from build123d import *

# Parameters (mm, degrees)
F0_W      = 90
F0_H      = 130
F1_DEPTH  = 20
F2_W      = 50
F2_H      = 2
F3_DEPTH  = 40
F4_W      = 50
F4_H      = 45
F5_DEPTH  = 2
F6_T      = -2
F7_R      = 2
F8_R      = 2
F9_R      = 2
F10_R     = 2
F11_R     = 2
F13_DEPTH = 25


# Not quite as in the source:
# - a shell that OpenCascade refuses in one call is made with other operations: the cavity is built on its own and cut out


with BuildPart() as f1:
    # F0 (on Top) → F1 (new body)
    with BuildSketch(Plane.XY):
        with Locations((45, -65)):
            Rectangle(F0_W, F0_H)
    extrude(amount=F1_DEPTH)

    # F2 (on face) → F3 (join)
    with BuildSketch(Plane(origin=(0, 0, 0), x_dir=(-1, 0, 0), z_dir=(0, 1, 0))):
        with Locations((-45, 1)):
            Rectangle(F2_W, F2_H)
    extrude(amount=F3_DEPTH)

    # F4 (on Top) → F5 (join)
    with BuildSketch(Plane.XY):
        Polygon((20, 40), (70, 40), (80, 40), (80, 105), (10, 105), (10, 40), align=None)
        with Locations((45, 72.5)):
            Rectangle(F4_W, F4_H, mode=Mode.SUBTRACT)
    extrude(amount=F5_DEPTH)

    # F6: a shell. OpenCascade refuses it in one call, so the cavity is built on its own and cut out:
    # the body offset inwards by the wall thickness, plus a prism from it out through each open face.
    f6_core = offset(f1.part, amount=F6_T, kind=Kind.INTERSECTION, mode=Mode.PRIVATE)
    f6_exits = [f6_core.faces().sort_by_distance(p)[0] for p in [
        (45, -2, 10),
    ]]
    add(f6_core, mode=Mode.SUBTRACT)
    extrude(f6_exits, amount=-F6_T, mode=Mode.SUBTRACT)

    # F7
    f7_edges = [f1.edges().sort_by_distance(p)[0] for p in [
        (0, -65, 20),
        (90, -65, 20),
        (90, -65, 0),
        (0, -65, 0),
    ]]
    fillet(f7_edges, radius=F7_R)

    # F8
    f8_edges = [f1.edges().sort_by_distance(p)[0] for p in [
        (45, -130, 0),
    ]]
    fillet(f8_edges, radius=F8_R)

    # F9
    f9_edges = [f1.edges().sort_by_distance(p)[0] for p in [
        (10, 40, 1),
        (10, 105, 1),
        (80, 105, 1),
        (80, 40, 1),
    ]]
    fillet(f9_edges, radius=F9_R)

    # F10
    f10_edges = [f1.edges().sort_by_distance(p)[0] for p in [
        (20, 40, 1),
        (70, 40, 1),
        (70, 0, 1),
        (20, 0, 1),
    ]]
    fillet(f10_edges, radius=F10_R)

    # F11
    f11_edges = [f1.edges().sort_by_distance(p)[0] for p in [
        (20, 50, 1),
        (20, 95, 1),
        (70, 50, 1),
        (70, 95, 1),
    ]]
    fillet(f11_edges, radius=F11_R)

    # F12 (on face) → F13 (cut)
    with BuildSketch(Plane.XZ.offset(130)):
        with BuildLine():
            Line((48.5, 14), (41.5, 14))
            ThreePointArc((41.5, 14), (37.5, 10), (41.5, 6))
            Line((41.5, 6), (48.5, 6))
            ThreePointArc((48.5, 6), (52.5, 10), (48.5, 14))
        make_face()
    extrude(amount=-F13_DEPTH, mode=Mode.SUBTRACT)


solid = f1.part
The model under review builds one solid part; all positions refer to its coordinate system, in mm. A direction names the side the tool comes from. Round coordinates to 2 decimals unless told otherwise and drop trailing zeros. Write each loop counter-clockwise with the first axis right and the second up, starting at its lowest first coordinate (ties: lowest second). Pieces come first, ordered by that corner, then holes. Notation, with made-up numbers: M 73.5,84.5 L 128.5,84.5 A24 ccw 128.5,122.5 Z; hole C 50,-16 d4. An arc over 180 degrees is marked long. Answer as CSV lines item,"result". Start each with the question number.
Q1. Consider section C-C, the plane y = -35. Give the boundary of the cut face in (x, z).
Q2. Consider section A-A, the plane z = 10. Give the boundary of the cut face in (x, y), then the cut area to 3 significant figures.
Q3. Tool access review of faces 1 (the face through (37.5, -129, 10.1)), 2 (the face through (90, -65, 10)), 3 (the face through (44, -128, 5)): name each direction out of +Z, -Z, +X, -X, +Y, -Y from which nothing blocks a thin tool from reaching the whole face with its end or side.
Q4. Clearance check with flat-ended pins moving along their axes: P1, Ø0.6, axis at x = 76, z = 1, coming from the -Y side; P2, Ø1, axis at y = 26, z = 1, coming from the -X side; P3, Ø0.6, axis at x = 45, y = -129, coming from the +Z side; P4, Ø1.6, axis at x = 16, z = 1.5, coming from the -Y side. State where each tip first meets the part, or that it passes through.
Q5. Wall thickness on line 1 along Z through (x, y) = (35, -82.5); line 2 along X through (y, z) = (-113, 3.25); line 3 along Y through (x, z) = (78, 10): over which ranges is each line inside the solid? List them lowest first.
Q6. Consider section D-D, the plane y = 65. Give the boundary of the cut face in (x, z).
Q7. Consider section B-B, the plane x = 27.5. Give the boundary of the cut face in (y, z).
Result set:
1,outline,"M 0,2 A2 ccw 2,0 L 88,0 A2 ccw 90,2 L 90,18 A2 ccw 88,20 L 2,20 A2 ccw 0,18 Z; hole M 2,2 L 88,2 L 88,18 L 2,18 Z"
2,outline,"M 0,-128 A2 ccw 2,-130 L 37.5,-130 L 37.5,-128 L 2,-128 L 2,0 L 0,0 Z; M 52.5,-130 L 88,-130 A2 ccw 90,-128 L 90,0 L 88,0 L 88,-128 L 52.5,-128 Z"
2,area,"660 mm²"
3,face 1,"+Y, -Y"
3,face 2,"+Z, -Z, +X, +Y, -Y"
3,face 3,"+Y"
4,P1,"stops at y = -129.87"
4,P2,"stops at x = 20"
4,P3,"stops at z = 19.87"
4,P4,"stops at y = -130"
5,line 1,"z = 0 to 2, 18 to 20"
5,line 2,"x = 0 to 2, 88 to 90"
5,line 3,"y = -130 to -128"
6,outline,"M 10,0 L 20,0 L 20,2 L 10,2 Z; M 70,0 L 80,0 L 80,2 L 70,2 Z"
7,outline,"M -130,2 A2 ccw -128,0 L 50,0 L 50,2 L -128,2 L -128,18 L 0,18 L 0,20 L -128,20 A2 ccw -130,18 Z; M 95,0 L 105,0 L 105,2 L 95,2 Z"
